Model file for the job. Use its own axes, mm. A direction names the side the tool comes from. Coordinates: 2 decimals unless noted, no trailing zeros. Write each loop counter-clockwise with the first axis right and the second up, starting at its lowest first coordinate (ties: lowest second). Pieces come first, ordered by that corner, then holes.
Q1. Pull direction Y, two halves, no side cores. Call faces 5 (the conical face through (-0.799, 2.537, 5.16)), 6 (the flat face through (0, 8, 3)), 7 (the flat face through (0, -4, 0)): released by +Y, released by -Y, zero draft, split by the parting line, or undercut.
Q2. Band-saw the part on C-C, the plane y = -4.5. Write the cut outline in (x, z), plus the area to 3 significant figures.
Q3. Which spindle directions (+Z, -Z, +X, -X, +Y, -Y) get a long thin tool onto all of the face, cutting with end or side? Do faces 1 (the flat face through (-0.493, 5.424, 5.706)), 2 (the flat face through (6, 0, 4.1)), 3 (the flat face through (-8, 0, 3)), 4 (the flat face through (-4, 0, 5)). Say none if no direction does.
Q4. Drill centre lines: probe 1 along Y at (x, z) = (0, 2.4); probe 2 along Z at (x, y) = (-4.75, 3); probe 3 along X at (y, z) = (6, 5). Where is each one in solid material? Low to high.
Q5. Band-saw the part on A-A, the plane y = 0. Write the cut outline in (x, z).
Q6. Band-saw the part on B-B, the plane z = 3. Write the cut outline in (x, y), plus the area to 3 significant figures.
Q7. Band-saw the part on D-D, the plane x = 6. Write the cut outline in (y, z), plus the area to 3 significant figures.
Q8. Pin check, flat tips, straight feed: P1, Ø2.5, axis at x = 6, y = 2.5, coming from the +Z side; P2, Ø1, axis at x = -6, y = -1.5, coming from the -Z side; P3, Ø4, axis at x = 0, y = 0, coming from the -Z side; P4, Ø1.4, axis at y = 3.5, z = 5, coming from the -X side. Stop position of each tip, or through.
from build123d import *

# Parameters (mm, degrees)
PAD_DEPTH   = 8
SKETCH001_R = 2.5
HOLE_DEPTH  = 6.001


with BuildPart() as part:
    # Sketch → Pad (new body, symmetric)
    with BuildSketch(Plane.XZ):
        with BuildLine():
            Line((-1, 6), (-3.7, 6))
            ThreePointArc((-3.7, 6), (-3.912132, 5.912132), (-4, 5.7))
            Line((-4, 5.7), (-4, 4.4))
            ThreePointArc((-4.3, 4.1), (-4.087868, 4.187868), (-4, 4.4))
            Line((-4.3, 4.1), (-7.7, 4.1))
            ThreePointArc((-7.7, 4.1), (-7.912132, 4.012132), (-8, 3.8))
            Line((-8, 3.8), (-8, 2.624264))
            ThreePointArc((-8, 2.624264), (-7.977164, 2.509459), (-7.912132, 2.412132))
            Line((-7.912132, 2.412132), (-5.587868, 0.087868))
            ThreePointArc((-5.587868, 0.087868), (-5.490541, 0.022836), (-5.375736, 0))
            Line((-5.375736, 0), (5.375736, 0))
            ThreePointArc((5.375736, 0), (5.490541, 0.022836), (5.587868, 0.087868))
            Line((5.587868, 0.087868), (7.912132, 2.412132))
            ThreePointArc((7.912132, 2.412132), (7.977164, 2.509459), (8, 2.624264))
            Line((8, 2.624264), (8, 3.8))
            ThreePointArc((8, 3.8), (7.912132, 4.012132), (7.7, 4.1))
            Line((7.7, 4.1), (4.3, 4.1))
            ThreePointArc((4, 4.4), (4.087868, 4.187868), (4.3, 4.1))
            Line((4, 4.4), (4, 5.7))
            ThreePointArc((4, 5.7), (3.912132, 5.912132), (3.7, 6))
            Line((3.7, 6), (1, 6))
            Line((1, 6), (0, 5.42))
            Line((0, 5.42), (-1, 6))
        make_face()
    extrude(amount=PAD_DEPTH, both=True)

    # Sketch001 → Hole (cut, through all)
    with BuildSketch(Plane.XY.offset(6)):
        Circle(SKETCH001_R)
    extrude(amount=-HOLE_DEPTH, mode=Mode.SUBTRACT)

    # Sketch002 → Groove (revolve, cut)
    with BuildSketch(Plane.YZ):
        Polygon((2.5, 6), (3.5, 6), (2.5, 5), align=None)
        Polygon((2.5, 0), (2.5, 1), (3.5, 0), align=None)
    revolve(axis=Axis((0, 0, 0), (0, 0, 1)), mode=Mode.SUBTRACT)


solid = part.part
Answer sheet:
1. face 5: undercut
1. face 6: released by +Y
1. face 7: zero draft
2. outline: (-8, 2.62) arc R0.3 ccw to (-7.91, 2.41) - (-5.59, 0.09) arc R0.3 ccw to (-5.38, 0) - (5.38, 0) arc R0.3 ccw to (5.59, 0.09) - (7.91, 2.41) arc R0.3 ccw to (8, 2.62) - (8, 3.8) arc R0.3 ccw to (7.7, 4.1) - (4.3, 4.1) arc R0.3 cw to (4, 4.4) - (4, 5.7) arc R0.3 ccw to (3.7, 6) - (1, 6) - (0, 5.42) - (-1, 6) - (-3.7, 6) arc R0.3 ccw to (-4, 5.7) - (-4, 4.4) arc R0.3 cw to (-4.3, 4.1) - (-7.7, 4.1) arc R0.3 ccw to (-8, 3.8) - close
2. area: 73.9 mm2
3. face 1: +Z, +Y, -Y
3. face 2: +Z, +X, +Y, -Y
3. face 3: +Z, -Z, -X, +Y, -Y
3. face 4: +Z, -X, +Y, -Y
4. probe 1: y = -8 to -2.5, 2.5 to 8
4. probe 2: z = 0 to 4.1
4. probe 3: x = -4 to 4
5. outline: (-8, 2.62) arc R0.3 ccw to (-7.91, 2.41) - (-5.59, 0.09) arc R0.3 ccw to (-5.38, 0) - (-3.5, 0) - (-2.5, 1) - (-2.5, 5) - (-3.5, 6) - (-3.7, 6) arc R0.3 ccw to (-4, 5.7) - (-4, 4.4) arc R0.3 cw to (-4.3, 4.1) - (-7.7, 4.1) arc R0.3 ccw to (-8, 3.8) - close; (2.5, 1) - (3.5, 0) - (5.38, 0) arc R0.3 ccw to (5.59, 0.09) - (7.91, 2.41) arc R0.3 ccw to (8, 2.62) - (8, 3.8) arc R0.3 ccw to (7.7, 4.1) - (4.3, 4.1) arc R0.3 cw to (4, 4.4) - (4, 5.7) arc R0.3 ccw to (3.7, 6) - (3.5, 6) - (2.5, 5) - close
6. outline: (-8, -8) - (8, -8) - (8, 8) - (-8, 8) - close; hole circle Ø5 at (0, 0)
6. area: 236 mm2
7. outline: (-8, 0.5) - (8, 0.5) - (8, 4.1) - (-8, 4.1) - close
7. area: 57.6 mm2
8. P1: stops at z = 4.1
8. P2: stops at z = 0.03
8. P3: passes through
8. P4: stops at x = -4.02
